Read the model definition and answer for the solid it produces. Units are mm, in the model's axes. A direction names the side the tool comes from. Coordinates: 2 decimals unless noted, no trailing zeros. Order: outer loops, then holes, each group sorted by start corner. A loop starts at its lowest first (then second) coordinate and runs counter-clockwise, first axis right, second up. Notation, with made-up numbers: (3, -5.75) -> (38, -5.75) arc R17 cw to (38, 26.25) -> close; hole circle Ø1 at (79.5, 15). An arc over 180 degrees is marked (long way). Return JSON: item names as keys, results as strings. Group by question number.
```python
from build123d import *

# Parameters (mm, degrees)
SKETCH1_W             = 12
SKETCH1_H             = 25
BOSS_EXTRUDE1_DEPTH   = 3
SKETCH1_3_W           = 5
SKETCH1_3_H           = 25
BOSS_EXTRUDE2_DEPTH   = 55
FILLET1_R             = 5
FILLET2_R             = 2
F_4_0MM_DOWEL_HOLE3_D = 4


with BuildPart() as part:
    # Sketch1 → Boss-Extrude1 (new body)
    with BuildSketch(Plane(origin=(0, 0, 0), x_dir=(1, 0, 0), z_dir=(0, 1, 0))):
        Rectangle(SKETCH1_W, SKETCH1_H)
    extrude(amount=BOSS_EXTRUDE1_DEPTH)

    # Sketch1<3> → Boss-Extrude2 (add)
    with BuildSketch(Plane(origin=(0, 0, 0), x_dir=(1, 0, 0), z_dir=(0, 1, 0))):
        with Locations((-8.5, 0)):
            Rectangle(SKETCH1_3_W, SKETCH1_3_H)
        with Locations((8.5, 0)):
            Rectangle(SKETCH1_3_W, SKETCH1_3_H)
    extrude(amount=BOSS_EXTRUDE2_DEPTH)

    # Fillet1
    fillet1_edges = [part.edges().sort_by_distance(p)[0] for p in [
        (-6, 3, 0),
        (-8.5, 55, 12.5),
        (-8.5, 55, -12.5),
        (8.5, 55, 12.5),
        (8.5, 55, -12.5),
        (6, 3, 0),
    ]]
    fillet(fillet1_edges, radius=FILLET1_R)

    # Fillet2
    fillet2_edges = [part.edges().sort_by_distance(p)[0] for p in [
        (11, 55, 0),
        (-11, 25, -12.5),
        (11, 25, -12.5),
        (11, 25, 12.5),
        (11, 53.535533906, 11.035533906),
        (11, 53.535533906, -11.035533906),
        (-11, 55, 0),
        (-11, 25, 12.5),
        (-11, 53.535533906, 11.035533906),
        (-11, 53.535533906, -11.035533906),
    ]]
    fillet(fillet2_edges, radius=FILLET2_R)

    # Ø4.0mm Dowel Hole3 (through all)
    with Locations(Plane.ZY.offset(11)):
        with Locations((0, 39.901131087)):
            Hole(F_4_0MM_DOWEL_HOLE3_D / 2)


solid = part.part
```
1. Find section C-C on z = -2.75. Determine the outline of the cut face in (x, y), and give its area (3 significant figures).
2. Which of the six approach directions +Z, -Z, +X, -X, +Y, -Y give full straight-line access (tool end or side, diameter ignored) to faces 5 (the face through (-8, 55, 0)), 6 (the face through (-5, 5, 0))?
3. Given pin 1 (12 mm diameter, centred on x = -5.5, z = 5.5, fed in from +Y); pin 2 (1 mm diameter, centred on x = 0, z = 4.5, fed in from +Y); pin 3 (3 mm diameter, centred on x = 3, z = 4.5, fed in from +Y), each flat-ended and moving along its own axis, determine where each tip first touches the part or whether it passes through.
4. Find section A-A on y = 36. Determine the outline of the cut face in (x, z).
5. Find section D-D on x = 4.25. Determine the outline of the cut face in (y, z).
6. Straight lines are drawn through the part: L1, parallel to X at y = 32, z = 3.5; L2, parallel to Y at x = -9.65, z = 0; L3, parallel to X at y = 42, z = 11.25. For each, find the intervals that lie inside material, in ascending order.
7. Find section B-B on z = 0. Determine the outline of the cut face in (x, y), and give its area (3 significant figures).
8. For a pull along X with two mould halves and no side action, classify faces 1 (the face through (6, 31, 0)), 2 (the face through (10.43, 24.65, -11.9)), 3 (the face through (-11, 26, 0)), 4 (the face through (-7.48, 53.57, 11)) as released by +X, released by -X, zero draft, split by the parting line, or undercut.
Result:
{
 "1": {"outline": "(-11, 0) -> (11, 0) -> (11, 53) arc R2 ccw to (9, 55) -> (6, 55) -> (6, 8) arc R5 cw to (1, 3) -> (-1, 3) arc R5 cw to (-6, 8) -> (-6, 55) -> (-9, 55) arc R2 ccw to (-11, 53) -> close", "area": "595 mm^2"},
 "2": {"face 5": "+Z, -Z, +X, -X, +Y", "face 6": "+Z, -Z, +Y"},
 "3": {"pin 1": "y = 55", "pin 2": "y = 3", "pin 3": "y = 4.43"},
 "4": {"outline": "(-11, -10.5) arc R2 ccw to (-9, -12.5) -> (-6, -12.5) -> (-6, 12.5) -> (-9, 12.5) arc R2 ccw to (-11, 10.5) -> close; (6, -12.5) -> (9, -12.5) arc R2 ccw to (11, -10.5) -> (11, 10.5) arc R2 ccw to (9, 12.5) -> (6, 12.5) -> close"},
 "5": {"outline": "(0, -12.5) -> (4.2, -12.5) -> (4.2, 12.5) -> (0, 12.5) -> close"},
 "6": {"L1": "-11 to -6, 6 to 11", "L2": "0 to 37.9, 41.9 to 54.89", "L3": "-10.85 to -6, 6 to 10.85"},
 "7": {"outline": "(-11, 0) -> (11, 0) -> (11, 37.9) -> (6, 37.9) -> (6, 8) arc R5 cw to (1, 3) -> (-1, 3) arc R5 cw to (-6, 8) -> (-6, 37.9) -> (-11, 37.9) -> close; (-11, 41.9) -> (-6, 41.9) -> (-6, 55) -> (-9, 55) arc R2 ccw to (-11, 53) -> close; (6, 41.9) -> (11, 41.9) -> (11, 53) arc R2 ccw to (9, 55) -> (6, 55) -> close", "area": "555 mm^2"},
 "8": {"face 1": "undercut", "face 2": "released by +X", "face 3": "released by -X", "face 4": "zero draft"}
}
